from build123d import *

# Parameters (mm, degrees)
SKETCH_W            = 16
SKETCH_H            = 8
PAD_DEPTH           = 2
SKETCH001_W         = 3
SKETCH001_H         = 8
PAD001_DEPTH        = 10
SKETCH002_R         = 1.1
HOLE_DEPTH          = 16.001
HOLE001_D           = 3.2
HOLE001_CSINK_D     = 5
HOLE001_CSINK_ANGLE = 90


with BuildPart() as part:
    # Sketch → Pad (new body)
    with BuildSketch(Plane.XY):
        Rectangle(SKETCH_W, SKETCH_H)
    extrude(amount=PAD_DEPTH)

    # Sketch001 (on Face6 of Pad) → Pad001 (join)
    with BuildSketch(Plane.XY.offset(2)):
        with Locations((-6.5, 0)):
            Rectangle(SKETCH001_W, SKETCH001_H)
        with Locations((6.5, 0)):
            Rectangle(SKETCH001_W, SKETCH001_H)
    extrude(amount=PAD001_DEPTH)

    # Sketch002 (on Face10 of Pad001) → Hole (cut, through all)
    with BuildSketch(Plane.YZ.offset(8)):
        with Locations((0, 8.2)):
            Circle(SKETCH002_R)
    extrude(amount=-HOLE_DEPTH, mode=Mode.SUBTRACT)

    # Hole001 (through all)
    with Locations(Plane.XY.offset(2)):
        with Locations((0, 0)):
            CounterSinkHole(HOLE001_D / 2, HOLE001_CSINK_D / 2, counter_sink_angle=HOLE001_CSINK_ANGLE)


solid = part.part
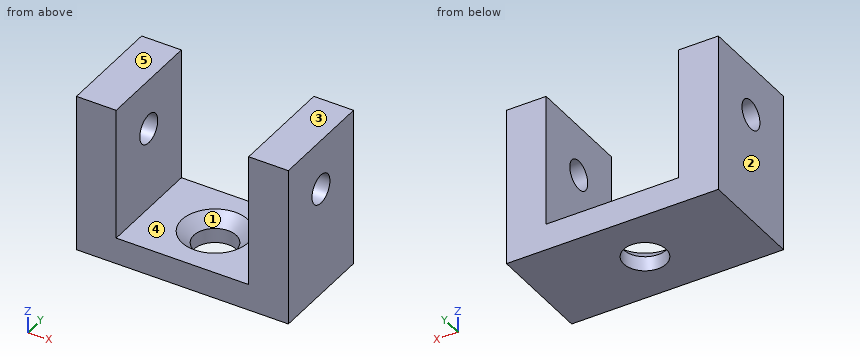
Input: part model. Units: mm. Frame: model coordinates. Face numbers are marked on the shaded views. A direction names the side the tool comes from. Give positions to 0.01 mm unless a question says otherwise; leave off trailing zeros. Order: outer loops, then holes, each group sorted by start corner. A loop starts at its lowest first (then second) coordinate and runs counter-clockwise, first axis right, second up. Notation, with made-up numbers: M 75,82 L 87,82 A22 cw 87,108 Z; hole C -38,-11 d1. An arc over 180 degrees is marked long. Answer as a JSON object with one key per item and string values.
1. Pull-direction query (X, two-part tool) for the marked faces 1, 2 and 3; classes: +X half, -X half, draft (parallel to the pull), parting line (faces both ways), or undercut.
Result sheet:
{"face 1": "undercut", "face 2": "-X half", "face 3": "draft"}
2. Cut plane D-D, the plane z = 4. Output: boundary loops of the cut face in (x, y).
Result sheet:
{"outline": "M -8,-4 L -5,-4 L -5,4 L -8,4 Z; M 5,-4 L 8,-4 L 8,4 L 5,4 Z"}
3. Cut plane C-C, the plane z = 8.2. Output: boundary loops of the cut face in (x, y).
Result sheet:
{"outline": "M -8,-4 L -5,-4 L -5,-1.1 L -8,-1.1 Z; M -8,1.1 L -5,1.1 L -5,4 L -8,4 Z; M 5,-4 L 8,-4 L 8,-1.1 L 5,-1.1 Z; M 5,1.1 L 8,1.1 L 8,4 L 5,4 Z"}
4. Ray query, line 1 (X direction, y = -1.5, z = 6.75); line 2 (X direction, y = 0, z = 0.3); line 3 (Z direction, x = -6.7, y = 0). Return the intervals inside material, ascending. Write a range as [from, to].
Result sheet:
{"line 1": "[-8, -5], [5, 8]", "line 2": "[-8, -1.6], [1.6, 8]", "line 3": "[0, 7.1], [9.3, 12]"}
5. Reachability of the marked faces 4 and 5 from +Z, -Z, +X, -X, +Y, -Y: full face, straight path, thin tool, end or side. Return the list, or none.
Result sheet:
{"face 4": "+Z, +Y, -Y", "face 5": "+Z, +X, -X, +Y, -Y"}
6. Cut plane A-A, the plane x = 0. Output: boundary loops of the cut face in (y, z), and give its area (3 significant figures).
Result sheet:
{"outline": "M -4,0 L -1.6,0 L -1.6,1.1 L -2.5,2 L -4,2 Z; M 1.6,0 L 4,0 L 4,2 L 2.5,2 L 1.6,1.1 Z", "area": "8.79 mm²"}
7. Cut plane B-B, the plane y = 0. Output: boundary loops of the cut face in (x, z), and give its area (3 significant figures).
Result sheet:
{"outline": "M -8,0 L -1.6,0 L -1.6,1.1 L -2.5,2 L -5,2 L -5,7.1 L -8,7.1 Z; M -8,9.3 L -5,9.3 L -5,12 L -8,12 Z; M 1.6,0 L 8,0 L 8,7.1 L 5,7.1 L 5,2 L 2.5,2 L 1.6,1.1 Z; M 5,9.3 L 8,9.3 L 8,12 L 5,12 Z", "area": "71.6 mm²"}
8. First-contact query: P1, Ø2.5, axis at x = -2, y = 0, coming from the +Z side. Flat tip, straight axial feed; report the tip coordinate or a pass-through.
Result sheet:
{"P1": "z = 2"}
